```python
from build123d import *

# Parameters (mm, degrees)
F0_R     = 11
F1_DEPTH = 6.35


# Not quite as in the source:
# - a length typed as a fraction of an inch, garbled in the dataset ("3 / 203.2 mm" for 3/8 in), is restored


with BuildPart() as f1:
    # F0 (on Front) → F1 (new body)
    with BuildSketch(Plane.XZ):
        with BuildLine():
            ThreePointArc((5.4528368022, -13.9737815501), (12.3853250267, -8.4618983676), (15, 0))
            ThreePointArc((15, 0), (14.956955291, 1.1355564373), (14.8280682104, 2.2645955817))
            ThreePointArc((14.8280682104, 2.2645955817), (14.5670313108, 3.5779321946), (14.1899117897, 4.8627567696))
            ThreePointArc((14.1899117897, 4.8627567696), (12.9903810568, 7.5), (11.3062267898, 9.8574457025))
            ThreePointArc((11.3062267898, 9.8574457025), (10.382095829, 10.8264530756), (9.3752314082, 11.7091859684))
            ThreePointArc((9.3752314082, 11.7091859684), (0, 15), (-9.3752314082, 11.7091859684))
            ThreePointArc((-9.3752314082, 11.7091859684), (-10.382095829, 10.8264530756), (-11.3062267898, 9.8574457025))
            ThreePointArc((-11.3062267898, 9.8574457025), (-12.9903810568, 7.5), (-14.1899117897, 4.8627567696))
            ThreePointArc((-14.1899117897, 4.8627567696), (-14.5670313108, 3.5779321946), (-14.8280682104, 2.2645955817))
            ThreePointArc((-14.8280682104, 2.2645955817), (-12.9903810568, -7.5), (-5.4528368022, -13.9737815501))
            ThreePointArc((-5.4528368022, -13.9737815501), (-4.1849354819, -14.4043852702), (-2.883685, -14.7202024721))
            ThreePointArc((-2.883685, -14.7202024721), (0, -15), (2.883685, -14.7202024721))
            ThreePointArc((2.883685, -14.7202024721), (4.1849354819, -14.4043852702), (5.4528368022, -13.9737815501))
        make_face()
        Circle(F0_R, mode=Mode.SUBTRACT)
        with BuildLine():
            ThreePointArc((14.1899117897, 4.8627567696), (14.5670313108, 3.5779321946), (14.8280682104, 2.2645955817))
            ThreePointArc((14.8280682104, 2.2645955817), (18.0862095917, 1.1045798418), (20.7543499599, -1.0959084571))
            ThreePointArc((20.7543499599, -1.0959084571), (22.0334229862, -0.6684079546), (23.3457232771, -0.3575182103))
            ThreePointArc((23.3457232771, -0.3575182103), (19.3449005461, 3.2647619918), (14.1899117897, 4.8627567696))
        make_face()
        with BuildLine():
            ThreePointArc((11.326259544, -17.4258400757), (8.0865105924, -16.2154068855), (5.4528368022, -13.9737815501))
            ThreePointArc((5.4528368022, -13.9737815501), (4.1849354819, -14.4043852702), (2.883685, -14.7202024721))
            ThreePointArc((2.883685, -14.7202024722), (6.8450834508, -18.3855563025), (11.982481491, -20.0392303225))
            ThreePointArc((11.982481491, -20.0392303225), (11.5955697619, -18.7473000611), (11.326259544, -17.4258400757))
        make_face()
        with BuildLine():
            ThreePointArc((23.3457232771, -0.3575182103), (22.0334229862, -0.6684079546), (20.7543499599, -1.0959084571))
            ThreePointArc((20.7543499599, -1.0959084571), (13.153553406, -7.5942075998), (11.326259544, -17.4258400757))
            ThreePointArc((11.326259544, -17.4258400757), (11.5955697619, -18.7473000611), (11.982481491, -20.0392303225))
            ThreePointArc((11.982481491, -20.0392303225), (28.6517428111, -29.8830850855), (41.1439344628, -15.0942075998))
            ThreePointArc((41.1439344628, -15.0942075998), (35.7101989431, -3.5405681778), (23.3457232771, -0.3575182103))
        make_face()
        with Locations((26.1439344628, -15.0942075998)):
            Circle(F0_R, mode=Mode.SUBTRACT)
        with BuildLine():
            ThreePointArc((9.3752314082, 11.7091859684), (10.382095829, 10.8264530756), (11.3062267898, 9.8574457025))
            ThreePointArc((11.3062267898, 9.8574457025), (12.4998170953, 15.1207943107), (11.3632417861, 20.3967485329))
            ThreePointArc((11.3632417861, 20.3967485329), (10.4378532243, 19.4157080157), (9.4280904158, 18.5217485329))
            ThreePointArc((9.4280904158, 18.5217485329), (9.9996989994, 15.1108270437), (9.3752314082, 11.7091859684))
        make_face()
        with BuildLine():
            ThreePointArc((-11.982481491, -20.0392303225), (-6.8450834508, -18.3855563025), (-2.883685, -14.7202024722))
            ThreePointArc((-2.883685, -14.7202024721), (-4.1849354819, -14.4043852702), (-5.4528368022, -13.9737815501))
            ThreePointArc((-5.4528368022, -13.9737815501), (-8.0865105924, -16.2154068855), (-11.326259544, -17.4258400757))
            ThreePointArc((-11.326259544, -17.4258400757), (-11.5955697619, -18.7473000611), (-11.982481491, -20.0392303225))
        make_face()
        with BuildLine():
            ThreePointArc((9.4280904158, 18.5217485329), (10.4378532243, 19.4157080157), (11.3632417861, 20.3967485329))
            ThreePointArc((11.3632417861, 20.3967485329), (14.0614477703, 24.9658021941), (15, 30.1884151995))
            ThreePointArc((15, 30.1884151995), (-5.2226130054, 44.2498629698), (-11.3632417861, 20.3967485329))
            ThreePointArc((-11.3632417861, 20.3967485329), (-10.4378532243, 19.4157080157), (-9.4280904158, 18.5217485329))
            ThreePointArc((-9.4280904158, 18.5217485329), (0, 15.1884151995), (9.4280904158, 18.5217485329))
        make_face()
        with Locations((0, 30.1884151995)):
            Circle(F0_R, mode=Mode.SUBTRACT)
        with BuildLine():
            ThreePointArc((-23.3457232771, -0.3575182103), (-39.1343155195, -22.5942075998), (-11.982481491, -20.0392303225))
            ThreePointArc((-11.982481491, -20.0392303225), (-11.5955697619, -18.7473000611), (-11.326259544, -17.4258400757))
            ThreePointArc((-11.326259544, -17.4258400757), (-11.1895851994, -16.2635826934), (-11.1439344628, -15.0942075998))
            ThreePointArc((-11.1439344628, -15.0942075998), (-13.7777756504, -6.6043244305), (-20.7543499599, -1.0959084571))
            ThreePointArc((-20.7543499599, -1.0959084571), (-22.0334229862, -0.6684079546), (-23.3457232771, -0.3575182103))
        make_face()
        with Locations((-26.1439344628, -15.0942075998)):
            Circle(F0_R, mode=Mode.SUBTRACT)
        with BuildLine():
            ThreePointArc((-11.3062267898, 9.8574457025), (-10.382095829, 10.8264530756), (-9.3752314082, 11.7091859684))
            ThreePointArc((-9.3752314082, 11.7091859684), (-9.9996989994, 15.1108270437), (-9.4280904158, 18.5217485329))
            ThreePointArc((-9.4280904158, 18.5217485329), (-10.4378532243, 19.4157080157), (-11.3632417861, 20.3967485329))
            ThreePointArc((-11.3632417861, 20.3967485329), (-12.4998170953, 15.1207943107), (-11.3062267898, 9.8574457025))
        make_face()
        with BuildLine():
            ThreePointArc((-20.7543499599, -1.0959084571), (-18.0862095917, 1.1045798418), (-14.8280682104, 2.2645955817))
            ThreePointArc((-14.8280682104, 2.2645955817), (-14.5670313108, 3.5779321946), (-14.1899117897, 4.8627567696))
            ThreePointArc((-14.1899117897, 4.8627567696), (-19.3449005461, 3.2647619918), (-23.3457232771, -0.3575182103))
            ThreePointArc((-23.3457232771, -0.3575182103), (-22.0334229862, -0.6684079546), (-20.7543499599, -1.0959084571))
        make_face()
    extrude(amount=-F1_DEPTH)


solid = f1.part
```
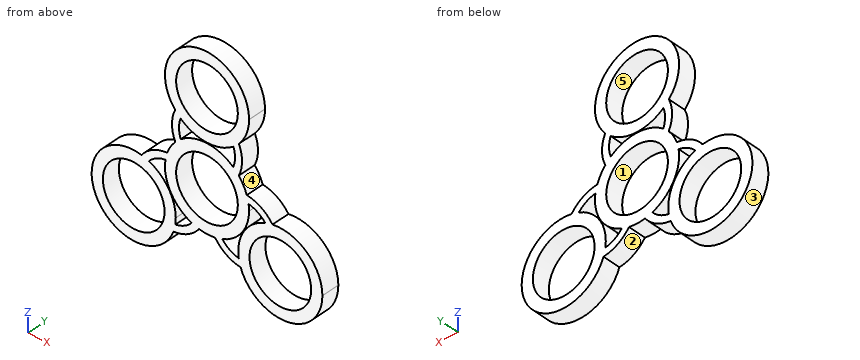
Geometry check sheet. Reference: the model listing, model coordinates, mm. Face numbers are marked on the shaded views. A direction names the side the tool comes from. Coordinates: 2 decimals unless noted, no trailing zeros. Write each loop counter-clockwise with the first axis right and the second up, starting at its lowest first coordinate (ties: lowest second). Pieces come first, ordered by that corner, then holes. Notation, with made-up numbers: M -25.75,56.5 L 11.25,56.5 A19 cw 11.25,72.5 Z; hole C 66,72 d2. An arc over 180 degrees is marked long. One line per item, written item: value. Start each with the question number.
(1) Scan lines: line 1 along Z through (x, y) = (-9, 5.75); line 2 along Z through (x, y) = (2, 4.25); line 3 along X through (y, z) = (4.25, 18). Record each from-to range of solid material in increasing order. Write a range as [from, to].
(2) Tool access check on the marked faces 4 and 5. Record the directions out of +Z, -Z, +X, -X, +Y, -Y that give a thin tool (end or side, any length) a straight path to the whole face; none if there is none.
(3) Sectioned sample at D-D, the plane y = 1.5. Enter the section's corners in (x, z).
(4) Sectioned sample at A-A, the plane x = 0. Enter the section's corners in (y, z).
(5) Sectioned sample at B-B, the plane x = 35. Enter the section's corners in (y, z).
(6) Release check for a two-part mould opening along Z. For the marked faces 1, 2 and 3 record: released by +Z, released by -Z, zero draft, split by the parting line, or undercut.
(7) Sectioned sample at C-C, the plane z = 28. Enter the section's corners in (x, y).
Filled sheet:
1. line 1: [-19.38, -16.69], [-12, -6.32], [6.32, 12], [18.19, 23.86], [36.51, 42.19]
1. line 2: [-14.87, -10.82], [10.82, 14.87], [15.32, 19.37], [41.01, 45.05]
1. line 3: [-12.18, -9.6], [-8.74, 8.74], [9.6, 12.18]
2. face 4: +X, +Y, -Y
2. face 5: +Y, -Y
3. outline: M -23.35,-0.36 A15 ccw long -11.98,-20.04 A12.5 ccw -2.88,-14.72 A15 ccw 2.88,-14.72 A12.5 ccw 11.98,-20.04 A15 ccw long 23.35,-0.36 A12.5 ccw 14.19,4.86 A15 ccw 11.31,9.86 A12.5 ccw 11.36,20.4 A15 ccw long -11.36,20.4 A12.5 ccw -11.31,9.86 A15 ccw -14.19,4.86 A12.5 ccw Z; hole C -26.14,-15.09 d22; hole M -20.75,-1.1 A15 cw -11.33,-17.43 A10 ccw -5.45,-13.97 A15 cw -14.83,2.26 A10 ccw Z; hole C 0,0 d22; hole C 0,30.19 d22; hole M -9.43,18.52 A10 ccw -9.38,11.71 A15 cw 9.38,11.71 A10 ccw 9.43,18.52 A15 cw Z; hole M 5.45,-13.97 A10 ccw 11.33,-17.43 A15 cw 20.75,-1.1 A10 ccw 14.83,2.26 A15 cw Z; hole C 26.14,-15.09 d22
4. outline: M 0,-15 L 6.35,-15 L 6.35,-11 L 0,-11 Z; M 0,11 L 6.35,11 L 6.35,15 L 0,15 Z; M 0,15.19 L 6.35,15.19 L 6.35,19.19 L 0,19.19 Z; M 0,41.19 L 6.35,41.19 L 6.35,45.19 L 0,45.19 Z
5. outline: M 0,-27.2 L 6.35,-27.2 L 6.35,-21.62 L 0,-21.62 Z; M 0,-8.57 L 6.35,-8.57 L 6.35,-2.99 L 0,-2.99 Z
6. face 1: undercut
6. face 2: released by -Z
6. face 3: split by the parting line
7. outline: M -14.84,0 L -10.78,0 L -10.78,6.35 L -14.84,6.35 Z; M 10.78,0 L 14.84,0 L 14.84,6.35 L 10.78,6.35 Z
